```python
from build123d import *

# Parameters (mm, degrees)
F0_R     = 4.5
F0_R_2   = 1.5
F1_DEPTH = 6
F2_R     = 2.5
F3_DEPTH = 20
F4_SIZE  = 0.5
F5_R     = 1.5
F6_DEPTH = 4.501


with BuildPart() as f1:
    # F0 (on Top) → F1 (new body, symmetric)
    with BuildSketch(Plane.XY):
        Circle(F0_R)
        Circle(F0_R_2, mode=Mode.SUBTRACT)
    extrude(amount=F1_DEPTH, both=True)

    # F2 (on face) → F3 (join)
    with BuildSketch(Plane.XY.offset(6)):
        Circle(F2_R)
    extrude(amount=F3_DEPTH)

    # F4
    f4_edges = [f1.edges().sort_by_distance(p)[0] for p in [
        (-2.5, 0, 26),
        (-4.5, 0, 6),
        (-1.5, 0, -6),
        (-4.5, 0, -6),
    ]]
    chamfer(f4_edges, length=F4_SIZE)

    # F5 (on Front) → F6 (cut, through all)
    with BuildSketch(Plane.XZ):
        Circle(F5_R)
    extrude(amount=-F6_DEPTH, mode=Mode.SUBTRACT)


solid = f1.part
```
Geometry check sheet. Reference: the model listing, model coordinates, mm. A direction names the side the tool comes from. Round coordinates to 2 decimals unless told otherwise and drop trailing zeros. Loops run counter-clockwise (first coordinate to the right, second up) from the corner with the lowest first, then second, coordinate; pieces in that order, holes last. Notation, with made-up numbers: (24.25, 5) - (31.25, 5) arc R30 cw to (31.25, 27) - close; hole circle Ø10 at (42.5, -25.5). An arc over 180 degrees is marked (long way). Use a Markdown table: item, result.
Q1. Material ranges on line 1 (Y direction, x = 0, z = 2.5); line 2 (Z direction, x = 0.5, y = -3); line 3 (X direction, y = -1.5, z = 23.5), recorded low to high.
Solutions:
| item | result |
|---|---|
| line 1 | y = -4.5 to -1.5, 1.5 to 4.5 |
| line 2 | z = -6 to 6 |
| line 3 | x = -2 to 2 |
Q2. Go/stop test with flat-tipped pins: P1, Ø3.5, axis at x = 0, y = 0, coming from the -Z side; P2, Ø3, axis at y = 1.5, z = 21, coming from the +X side; P3, Ø2.5, axis at x = 0, z = 0, coming from the +Y side; P4, Ø4, axis at x = -2, y = -1, coming from the +Z side. Record where each tip stops, or that it passes through.
Solutions:
| item | result |
|---|---|
| P1 | stops at z = -5.75 |
| P2 | stops at x = 2.5 |
| P3 | stops at y = -0.83 |
| P4 | stops at z = 26 |
Q3. Cross-section at A-A on x = 0. Record the cut outline in (y, z).
Solutions:
| item | result |
|---|---|
| outline | (-4.5, -5.5) - (-4, -6) - (-2, -6) - (-1.5, -5.5) - (-1.5, 6) - (1.5, 6) - (1.5, 1.5) - (4.5, 1.5) - (4.5, 5.5) - (4, 6) - (2.5, 6) - (2.5, 25.5) - (2, 26) - (-2, 26) - (-2.5, 25.5) - (-2.5, 6) - (-4, 6) - (-4.5, 5.5) - close; (1.5, -5.5) - (2, -6) - (4, -6) - (4.5, -5.5) - (4.5, -1.5) - (1.5, -1.5) - close |
Q4. Cross-section at B-B on z = 20. Record the cut outline in (x, y).
Solutions:
| item | result |
|---|---|
| outline | circle Ø5 at (0, 0) |
Q5. Draft check along Y on faces 1 (the flat face through (0, 0, 6)), 2 (the cylindrical face through (-0.54, -2.44, 15.61)), 3 (the flat face through (0, 0, 26)). Enter one of: released by +Y, released by -Y, zero draft, split by the parting line, or undercut.
Solutions:
| item | result |
|---|---|
| face 1 | undercut |
| face 2 | split by the parting line |
| face 3 | zero draft |
Q6. Access from +Z, -Z, +X, -X, +Y, -Y to the whole of each face (thin tool, end or side, straight path). Record for faces 4 (the cylindrical face through (-0.98, -4.39, 0.08)), 5 (the flat face through (-2, -1, -6)), 6 (the flat face through (-2, -2, 6)), 7 (the cylindrical face through (-1.5, 2.72, 0.07)), 8 (the cylindrical face through (-0.325, -1.464, 0.17)).
Solutions:
| item | result |
|---|---|
| face 4 | +Z, -Z |
| face 5 | -Z, +X, -X, +Y, -Y |
| face 6 | +Z |
| face 7 | +Y |
| face 8 | -Z |
Q7. Cross-section at C-C on z = 0. Record the cut outline in (x, y), plus the area to 3 significant figures.
Solutions:
| item | result |
|---|---|
| outline | (-1.5, 0) - (-1.5, 4.24) arc R4.5 ccw (long way) to (1.5, 4.24) - (1.5, 0) arc R1.5 cw to start |
| area | 46.8 mm2 |
